Read the model definition and answer for the solid it produces. Units are mm, in the model's axes. A direction names the side the tool comes from. Round coordinates to 2 decimals unless told otherwise and drop trailing zeros. Order: outer loops, then holes, each group sorted by start corner. A loop starts at its lowest first (then second) coordinate and runs counter-clockwise, first axis right, second up. Notation, with made-up numbers: (51.5, -31.75) -> (85.5, -31.75) arc R27 cw to (85.5, -1.75) -> close; hole circle Ø9 at (-4.5, -21.75). An arc over 180 degrees is marked (long way). Use a Markdown table: item, result. Add a question column.
1. Section C-C, the plane z = 0 is taken. Give the vertices of the cut face in (x, y).
2. For faces 4 (the face through (3, -8, 13)), 5 (the face through (10, 0, 3)), 6 (the face through (5, 2, -1.6)), determine the directions among +Z, -Z, +X, -X, +Y, -Y from which every point of the face is accessible in a straight line to the end or side of a thin tool.
3. Section D-D, the plane y = 7 is taken. Give the vertices of the cut face in (x, z), then the cut area to 3 significant figures.
4. The mould has two halves that part along Y. Classify faces 1 (the face through (0, 4, 0)), 2 (the face through (6.55, -12.65, 8.06)), 3 (the face through (5, 2, 1.6)): +Y half, -Y half, draft (parallel to the pull), parting line (faces both ways), or undercut.
5. Section A-A, the plane y = 0 is taken. Give the vertices of the cut face in (x, z).
6. Section B-B, the plane x = 3.75 is taken. Give the vertices of the cut face in (y, z), then the cut area to 3 significant figures.
7. Given pin 1 (2.5 mm diameter, centred on x = 6, z = -0.5, fed in from -Y); pin 2 (4 mm diameter, centred on x = 6.5, y = -10.5, fed in from +Z); pin 3 (1 mm diameter, centred on y = 10, z = -13, fed in from +X), each flat-ended and moving along its own axis, determine where each tip first touches the part or whether it passes through.
8. Consider L1, parallel to Y at x = 7.5, z = 0; L2, parallel to Y at x = 4.25, z = -11; L3, parallel to Z at x = 7.25, y = -9. Determine where each line is inside the solid, lowest interval first. Write a range as [from, to].
```python
from build123d import *

# Parameters (mm, degrees)
SKETCH2_R          = 1.5
CUT_EXTRUDE1_DEPTH = 27.69269563


with BuildPart() as part:
    # Sketch1 → Revolve1 (revolve)
    with BuildSketch(Plane.XY, mode=Mode.PRIVATE) as revolve1_sk:
        Polygon((0, 0), (0, 17.5), (3, 17.5), (3, 15), (10, 15), (10, 0), align=None)
    revolve(revolve1_sk.sketch.rotate(Axis((0, 0, 0), (1, 0, 0)), 90), axis=Axis((0, 0, 0), (1, 0, 0)))

    # Sketch2 → Cut-Extrude1 (cut, through all)
    with BuildSketch(Plane(origin=(10, 0, 0), x_dir=(0, 0, -1), z_dir=(1, 0, 0))):
        with Locations((-11, 0)):
            Circle(SKETCH2_R)
        with Locations(Location((11, 0, 0), (0, 0, 180))):
            Circle(SKETCH2_R)
        with BuildLine():
            Line((-1.6, 1.2), (-1.6, 2.2))
            Line((-1.6, 2.2), (1.6, 2.2))
            Line((1.6, 2.2), (1.6, 1.2))
            ThreePointArc((1.6, 1.2), (0, -2), (-1.6, 1.2))
        make_face()
    extrude(amount=-CUT_EXTRUDE1_DEPTH, mode=Mode.SUBTRACT)


solid = part.part
```
Verdict:
| question | item | result |
|---|---|---|
| 1 | outline | (0, -17.5) -> (3, -17.5) -> (3, -15) -> (10, -15) -> (10, -2) -> (0, -2) -> close; (0, 2.2) -> (10, 2.2) -> (10, 15) -> (3, 15) -> (3, 17.5) -> (0, 17.5) -> close |
| 2 | face 4 | +X |
| 2 | face 5 | +Z, -Z, +X, +Y, -Y |
| 2 | face 6 | +X, -X |
| 3 | outline | (0, -16.04) -> (3, -16.04) -> (3, -13.27) -> (10, -13.27) -> (10, 13.27) -> (3, 13.27) -> (3, 16.04) -> (0, 16.04) -> close |
| 3 | area | 282 mm2 |
| 4 | face 1 | draft |
| 4 | face 2 | parting line |
| 4 | face 3 | undercut |
| 5 | outline | (0, -17.5) -> (3, -17.5) -> (3, -15) -> (10, -15) -> (10, -12.5) -> (0, -12.5) -> close; (0, -9.5) -> (10, -9.5) -> (10, -2) -> (0, -2) -> close; (0, 2) -> (10, 2) -> (10, 9.5) -> (0, 9.5) -> close; (0, 12.5) -> (10, 12.5) -> (10, 15) -> (3, 15) -> (3, 17.5) -> (0, 17.5) -> close |
| 6 | outline | circle Ø30 at (0, 0); hole circle Ø3 at (0, -11); hole circle Ø3 at (0, 11); hole (1.2, -1.6) -> (2.2, -1.6) -> (2.2, 1.6) -> (1.2, 1.6) arc R2 ccw (long way) to start |
| 6 | area | 679 mm2 |
| 7 | pin 1 | stops at y = -15 |
| 7 | pin 2 | stops at z = 12.36 |
| 7 | pin 3 | stops at x = 3 |
| 8 | L1 | y = [-15, -2], [2.2, 15] |
| 8 | L2 | y = [-10.2, -1.5], [1.5, 10.2] |
| 8 | L3 | z = [-12, 12] |
